Answer from the drawing. Dimensions are ordinates in mm from the lowest x, y and z of the part. A direction names the side the tool comes from. Give positions to 0.01 mm unless a question says otherwise; leave off trailing zeros. Loops run counter-clockwise (first coordinate to the right, second up) from the corner with the lowest first, then second, coordinate; pieces in that order, holes last. Notation, with made-up numbers: (11, 77.5) - (56, 77.5) arc R20 ccw to (56, 114.5) - close; hole circle Ø3 at (0, 50). An arc over 180 degrees is marked (long way). Answer as CSV lines item,"result". Start each with the question number.
1) Flat-ended cylindrical pins translate along their axes: pin 1 (5 mm diameter, centred on x = 39, y = 43, fed in from +Z); pin 2 (1.5 mm diameter, centred on y = 10.5, z = 13.5, fed in from +X). Find the tip coordinate at first contact, or state that the pin passes through.
2) For the marked faces 1 and 2, determine the directions among +Z, -Z, +X, -X, +Y, -Y from which every point of the face is accessible in a straight line to the end or side of a thin tool.
3) A cutting plane is placed at A-A (z = 11.5). Determine the outline of the cut face in (x, y), and give its area (3 significant figures).
4) A cutting plane is placed at D-D (y = 6). Determine the outline of the cut face in (x, z).
5) For a pull along Y with two mould halves and no side action, classify the marked faces 3, 4, 5 and 6 as pulls with the +Y half, pulls with the -Y half, needs draft (parallel to the pull), parting line crosses it, or undercut.
6) A cutting plane is placed at B-B (y = 17). Determine the outline of the cut face in (x, z).
7) Find the intervals of material crossed by line 1 along Y through (x, z) = (59.5, 10.25); line 2 along X through (y, z) = (43, 17.5); line 3 along Z through (x, y) = (14, 4.5), in increasing order.
8) A cutting plane is placed at C-C (x = 22.5). Determine the outline of the cut face in (y, z).
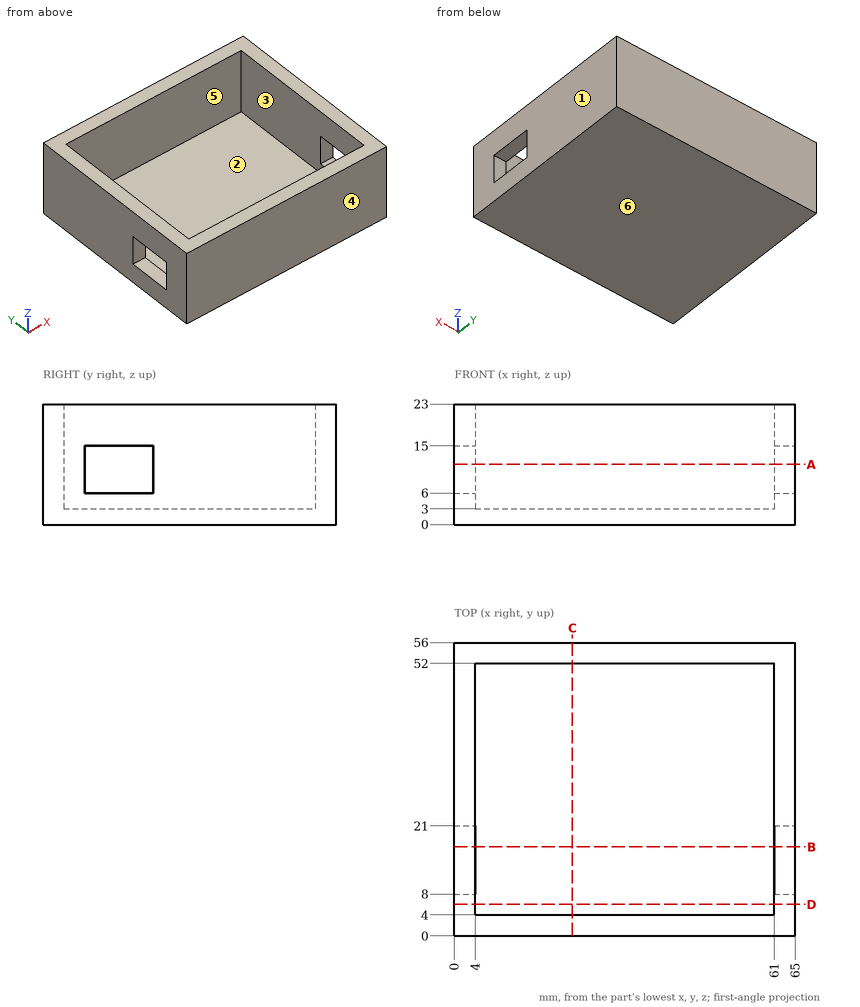
Ans:
1,pin 1,"z = 3"
1,pin 2,"through"
2,face 1,"+Z, -Z, +X, +Y, -Y"
2,face 2,"+Z"
3,outline,"(0, 0) - (65, 0) - (65, 8) - (61, 8) - (61, 4) - (4, 4) - (4, 8) - (0, 8) - close; (0, 21) - (4, 21) - (4, 52) - (61, 52) - (61, 21) - (65, 21) - (65, 56) - (0, 56) - close"
3,area,"800 mm2"
4,outline,"(0, 0) - (65, 0) - (65, 23) - (61, 23) - (61, 3) - (4, 3) - (4, 23) - (0, 23) - close"
5,face 3,"undercut"
5,face 4,"pulls with the -Y half"
5,face 5,"undercut"
5,face 6,"needs draft"
6,outline,"(0, 0) - (65, 0) - (65, 6) - (61, 6) - (61, 3) - (4, 3) - (4, 6) - (0, 6) - close; (0, 15) - (4, 15) - (4, 23) - (0, 23) - close; (61, 15) - (65, 15) - (65, 23) - (61, 23) - close"
7,line 1,"0 to 4, 52 to 56"
7,line 2,"0 to 4, 61 to 65"
7,line 3,"0 to 3"
8,outline,"(0, 0) - (56, 0) - (56, 23) - (52, 23) - (52, 3) - (4, 3) - (4, 23) - (0, 23) - close"
